Part model, mm, in its own coordinate system. Face numbers are marked on the shaded views. A direction names the side the tool comes from. Round coordinates to 2 decimals unless told otherwise and drop trailing zeros. Write each loop counter-clockwise with the first axis right and the second up, starting at its lowest first coordinate (ties: lowest second). Pieces come first, ordered by that corner, then holes.
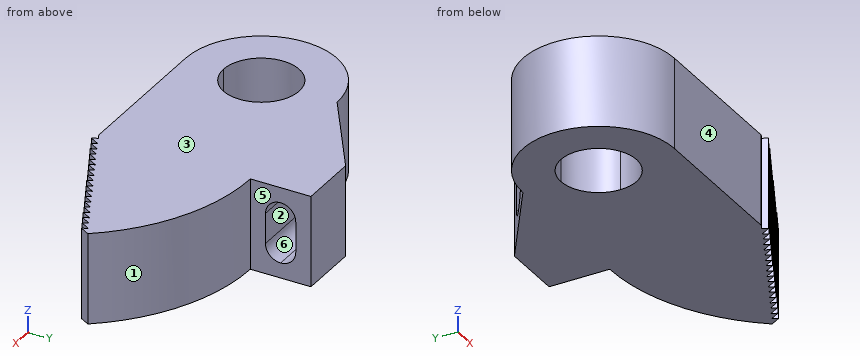
from build123d import *

# Parameters (mm, degrees)
F1_DEPTH = 7.62
F3_DEPTH = 7.62
F4_W     = 2.54
F4_H     = 2.54
F5_DEPTH = 25.4
F6_R     = 1.26999


# Not quite as in the source:
# - a fillet or chamfer is up to 0.001 mm smaller than in the source, because OpenCascade refuses the exact size


with BuildPart() as f1:
    # F0 (on Top) → F1 (new body)
    with BuildSketch(Plane.XY):
        with BuildLine():
            Line((-12.7, -6.35), (-12.7, 0))
            Line((-12.7, 0), (-19.05, 0))
            ThreePointArc((-19.05, 0), (-20.9098719395, -4.4901280605), (-25.4, -6.35))
            Line((-25.4, -6.35), (-12.7, -6.35))
        make_face()
        with BuildLine():
            Line((-12.7, 6.35), (-12.7, 0))
            Line((-12.7, 0), (-2.2980148465, 0))
            Line((-2.2980148465, 0), (-1.3816523133, 0.5641126772))
            Line((-1.3816523133, 0.5641126772), (0, 0))
            ThreePointArc((0, 0), (-5.6004841714, 4.6740316571), (-12.7, 6.35))
        make_face()
        with BuildLine():
            Line((-19.05, 0), (-12.7, 0))
            Line((-12.7, 0), (-12.7, 6.35))
            Line((-12.7, 6.35), (-25.4, 6.35))
            ThreePointArc((-25.4, 6.35), (-20.9098719395, 4.4901280605), (-19.05, 0))
        make_face()
        Polygon((-2.2980148465, 0), (-12.7, 0), (-12.7, -6.35), (-12.2375346417, -6.1187673209), align=None)
        with BuildLine():
            ThreePointArc((-25.4, -6.35), (-20.9098719395, -4.4901280605), (-19.05, 0))
            Line((-19.05, 0), (-22.225, 0))
            ThreePointArc((-22.225, 0), (-23.1549359697, -2.2450640303), (-25.4, -3.175))
            Line((-25.4, -3.175), (-25.4, -6.35))
        make_face()
        with BuildLine():
            Line((-22.225, 0), (-19.05, 0))
            ThreePointArc((-19.05, 0), (-20.9098719395, 4.4901280605), (-25.4, 6.35))
            Line((-25.4, 6.35), (-25.4, 3.175))
            ThreePointArc((-25.4, 3.175), (-23.1549359697, 2.2450640303), (-22.225, 0))
        make_face()
        Polygon((-1.3816523133, 0.5641126772), (-2.2980148465, 0), (0, 0), align=None)
        Polygon((0, 0), (-2.2980148465, 0), (-12.2375346417, -6.1187673209), (-0.6815535195, -0.3407767598), align=None)
        with BuildLine():
            Line((-25.4, 3.175), (-25.4, 6.35))
            ThreePointArc((-25.4, 6.35), (-31.75, 0), (-25.4, -6.35))
            Line((-25.4, -6.35), (-25.4, -3.175))
            ThreePointArc((-25.4, -3.175), (-28.575, 0), (-25.4, 3.175))
        make_face()
        Polygon((-0.454369013, -0.7951457728), (0, 0), (-0.6815535195, -0.3407767598), (-0.6815020435, -0.3408797119), align=None)
        Polygon((-0.6815535195, -0.3407767598), (-12.2375346417, -6.1187673209), (-12.2666181754, -6.1366711411), (-11.5850646558, -5.7958943813), (-11.3579903771, -6.2500430279), (-10.903621364, -5.4548972551), (-10.6765470852, -5.9090459018), (-10.2221780722, -5.113900129), (-9.9951037934, -5.5680487756), (-9.5407347804, -4.7729030028), (-9.3136605016, -5.2270516495), (-8.8592914886, -4.4319058767), (-8.6322172098, -4.8860545233), (-8.1778481968, -4.0909087505), (-7.950773918, -4.5450573971), (-7.496404905, -3.7499116243), (-7.2693306262, -4.204060271), (-6.8149616132, -3.4089144982), (-6.5878873344, -3.8630631448), (-6.1335183214, -3.067917372), (-5.9063852987, -3.5221834368), (-5.4520162857, -2.727037664), (-5.224883263, -3.1813037288), (-4.7705142499, -2.386157956), (-4.5433812273, -2.8404240208), (-4.0890122142, -2.045278248), (-3.8618791916, -2.4995443128), (-3.4075101785, -1.70439854), (-3.1803771559, -2.1586646048), (-2.7260081428, -1.363518832), (-2.4988751201, -1.8177848968), (-2.0445061071, -1.022639124), (-1.8173730844, -1.4769051888), (-1.3630040714, -0.681759416), (-1.1358710487, -1.1360254808), (-0.6815020357, -0.340879708), align=None)
        Polygon((-11.5850646558, -5.7958943813), (-12.2666181754, -6.1366711411), (-12.0394336689, -6.5910401541), align=None)
    extrude(amount=F1_DEPTH)

    # F2 (on face) → F3 (join)
    with BuildSketch(Plane.XY.offset(7.62)):
        Polygon((-25.4, 6.35), (-12.7, 6.35), (-12.7, 11.43), (-17.78, 11.43), align=None)
    extrude(amount=-F3_DEPTH)

    # F4 (on face) → F5 (cut)
    with BuildSketch(Plane.YZ.offset(-12.7)):
        with Locations((8.89, 2.54)):
            Rectangle(F4_W, F4_H)
        with Locations((8.89, 5.08)):
            Rectangle(F4_W, F4_H)
    extrude(amount=-F5_DEPTH, mode=Mode.SUBTRACT)

    # F6 (radius 1.27 in the source; OpenCascade refuses exactly that, so slightly less here)
    f6_edges = [f1.edges().sort_by_distance(p)[0] for p in [
        (-18.0975, 7.62, 1.27),
        (-18.0975, 7.62, 6.35),
        (-16.1925, 10.16, 6.35),
        (-16.1925, 10.16, 1.27),
    ]]
    fillet(f6_edges, radius=F6_R)


solid = f1.part
Q1. Saw through at B-B, the plane y = 8.25. Write the cut outline in (x, z).
Q2. Saw through at C-C, the plane z = 4.75. Give the number of separate pieces and of enclosed holes in the cut face, and give its area (3 significant figures).
Q3. Tool access for the marked faces 4, 5 and 6: list every direction of +Z, -Z, +X, -X, +Y, -Y with a clear straight run to the whole face (end or side of a thin tool).
Q4. Wall check: line 1 (Y direction, x = -13, z = 4.5); line 2 (X direction, y = -2, z = 5.75); line 3 (Y direction, x = -14, z = 0.75). Give the ranges that are in metal, low to high.
Q5. Drop flat-ended pins along their axis: P1, Ø4, axis at y = 6, z = 4, coming from the +X side; P2, Ø4, axis at y = 8.5, z = 2.5, coming from the +X side; P3, Ø2, axis at x = -16, z = 4, coming from the -Y side. Give the stop position or say it passes through.
Q6. Two-plate mould, pull along Z, no slides. Class the marked faces 1, 2 and 3: released by +Z, released by -Z, zero draft, split by the parting line, or undercut.
Q7. Saw through at D-D, the plane x = -26.5. Write the cut outline in (y, z).
Computed:
1. outline: (-22.55, 0) - (-12.7, 0) - (-12.7, 1.44) - (-22.55, 1.44) - close; (-22.55, 6.18) - (-12.7, 6.18) - (-12.7, 7.62) - (-22.55, 7.62) - close
2. separate pieces: 2
2. enclosed holes: 1
2. area: 316 mm2
3. face 4: +Z, -Z, -X, -Y
3. face 5: +Z, -Z, +X, +Y
3. face 6: +X, -X
4. line 1: y = -6.35 to 7.62, 10.16 to 11.43
4. line 2: x = -31.43 to -27.87, -22.93 to -3.58, -3.26 to -3.09
4. line 3: y = -6.35 to 11.43
5. P1: stops at x = -4.39
5. P2: stops at x = -12.7
5. P3: stops at y = -6.35
6. face 1: zero draft
6. face 2: undercut
6. face 3: released by +Z
7. outline: (-6.25, 0) - (-2.98, 0) - (-2.98, 7.62) - (-6.25, 7.62) - close; (2.98, 0) - (6.25, 0) - (6.25, 7.62) - (2.98, 7.62) - close
